Autodesk Inventor part; units mm, degrees
ref_plane "YZ Plane" through (0, 0, 0) normal (1, 0, 0) x (0, 1, 0)
ref_plane "XZ Plane" through (0, 0, 0) normal (0, 1, 0) x (-1, 0, 0)
ref_plane "XY Plane" through (0, 0, 0) normal (0, 0, 1) x (1, 0, 0)
sketch "Sketch1" plane through (0, 0, 0) normal (0, 0, 1) x (1, 0, 0)
  line L0 (0, 0) -> (25.4, 0)
  line L1 (25.4, 0) -> (25.4, 25.4)
  line L2 (25.4, 25.4) -> (0, 25.4)
  line L3 (0, 25.4) -> (0, 0)
  line L4 (3.175, 3.175) -> (22.225, 3.175)
  line L5 (22.225, 3.175) -> (22.225, 22.225)
  line L6 (22.225, 22.225) -> (3.175, 22.225)
  line L7 (3.175, 22.225) -> (3.175, 3.175)
  dimension "d0" = 25.4
  dimension "d1" = 25.4
  dimension "d2" = 19.05
  dimension "d3" = 19.05
  dimension "d4" = 3.175
  dimension "d5" = 3.175
extrude "Extrusion1" add sketch "Sketch1" along normal blind 657.225
sketch "Sketch2" plane through (0, 25.4, 0) normal (0, 1, 0) x (1, 0, 0)
  line L0 (25.4, 0) -> (0, 0)
  line L1 (0, 0) -> (0, -657.225)
  point P0 (12.7, -12.7)
  point P1 (12.7, -139.7)
  dimension "d8" = 12.7
  dimension "d9" = 12.7
  dimension "d10" = 12.7
  dimension "d11" = 139.7
hole "Hole1" at (12.7, 25.4, 12.7) at (12.7, 25.4, 139.7) direction (0, -1, 0) diameter 6.35 end through all
sketch "Sketch3" plane through (0, 0, 0) normal (-1, 0, 0) x (0, 0, 1)
  line L0 (0, 0) -> (657.225, 0)
  line L1 (657.225, 25.4) -> (657.225, 0)
  point P0 (644.525, 12.7)
  point P1 (619.125, 12.7)
  point P2 (406.4, 12.7)
  point P3 (381, 12.7)
  dimension "d19" = 12.7
  dimension "d20" = 12.7
  dimension "d21" = 12.7
  dimension "d22" = 25.4
  dimension "d23" = 212.725
  dimension "d24" = 12.7
  dimension "d25" = 12.7
  dimension "d26" = 25.4
hole "Hole2" at (0, 12.7, 644.525) at (0, 12.7, 619.125) at (0, 12.7, 406.4) at (0, 12.7, 381) direction (1, 0, 0) diameter 6.35 end through all
sketch "Sketch5" plane through (0, 25.4, 0) normal (0, 1, 0) x (1, 0, 0)
  circle A0 centre (12.7, -12.7) radius 3.175
  circle A1 centre (12.7, -139.7) radius 3.175
  line L0 (25.4, 0) -> (0, 0)
  line L1 (0, 0) -> (0, -657.225)
  line L2 (25.4, -657.225) -> (0, -657.225)
  line L3 (25.4, 0) -> (25.4, -657.225)
  line L4 (0, -657.225) -> (22.225, -657.225)
  line L5 (22.225, -657.225) -> (3.175, -657.225)
  line L6 (0, -657.225) -> (0, -606.425)
  line L7 (0, 0) -> (0, -657.225)
  line L8 (0, -606.425) -> (22.225, -657.225)
  dimension "d37" = 22.225
  dimension "d38" = 50.8
extrude "Extrusion3" cut sketch "Sketch5" against normal blind 25.4 contours L8 L2 L1
sketch "Sketch6" plane through (25.4, 0, 0) normal (1, 0, 0) x (0, 0, -1)
  line L0 (0, 25.4) -> (-657.225, 25.4)
  line L1 (-657.225, 0) -> (-657.225, 25.4)
  point P0 (-593.725, 12.7)
  point P1 (-514.35, 12.7)
  point P2 (-434.975, 12.7)
  dimension "d41" = 12.7
  dimension "d42" = 63.5
  dimension "d43" = 142.875
  dimension "d44" = 12.7
  dimension "d45" = 12.7
  dimension "d46" = 222.25
hole "Hole3" at (25.4, 12.7, 593.725) at (25.4, 12.7, 514.35) at (25.4, 12.7, 434.975) direction (-1, 0, 0) diameter 6.35 end through all
properties part number "pickup arm 1x1 long" material "Aluminum 6061"
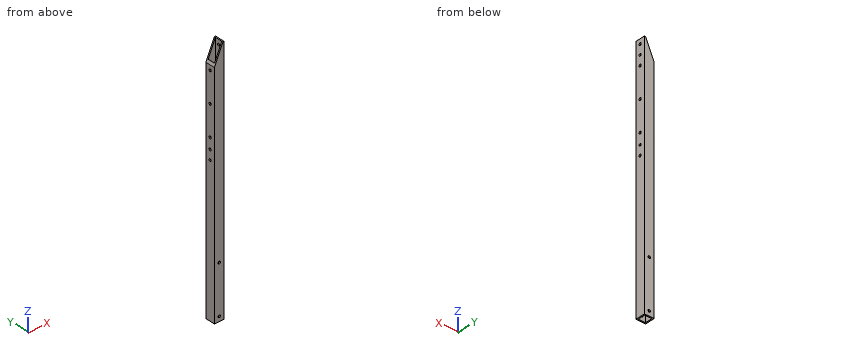
Geometry check sheet. Reference: the model listing, model coordinates, mm. Round coordinates to 2 decimals unless told otherwise and drop trailing zeros. Order: outer loops, then holes, each group sorted by start corner. A loop starts at its lowest first (then second) coordinate and runs counter-clockwise, first axis right, second up. Notation, with made-up numbers: M -34,7.5 L -5,7.5 A21 cw -5,44.5 Z; hole C 74,72 d3. An arc over 180 degrees is marked long. Answer in a Markdown table with one row per item. Add a question column.
Item 1: Depth check by flat-ended pin: pin 1 Ø10 at (y, z) = (12.7, 644.525) entering from -X (3 decimals); pin 2 Ø10 at (x, y) = (16, 3) entering from +Z (3 decimals). Enter the tip coordinate at first touch or a pass-through.
Item 2: Sectioned sample at A-A, the plane z = 113.5. Enter the section's corners in (x, y) (3 decimals), plus the area to 3 significant figures.
Item 3: Material ranges on L1, parallel to X at y = 20.5, z = 363 (3 decimals); L2, parallel to X at y = 24, z = 12.7 (3 decimals), recorded low to high. Write a range as [from, to].
Filled in:
| question | item | result |
|---|---|---|
| 1 | pin 1 | stops at x = 22.225 |
| 1 | pin 2 | stops at z = 654.425 |
| 2 | outline | M 0,0 L 25.4,0 L 25.4,25.4 L 0,25.4 Z; hole M 3.175,3.175 L 22.225,3.175 L 22.225,22.225 L 3.175,22.225 Z |
| 2 | area | 282 mm² |
| 3 | L1 | x = [0, 3.175], [22.225, 25.4] |
| 3 | L2 | x = [0, 9.525], [15.875, 25.4] |
